Solid Edge part; units mm, degrees
sketch "Sketch1" plane through (0, 0, 0) normal (0, 0, 1) x (1, 0, 0)
  circle A0 centre (0, 0) radius 3.5
extrude "Protrusion1" add sketch "Sketch1" along normal blind 4
sketch "Sketch2" plane through (0, 0, 0) normal (0, 0, -1) x (1, 0, 0)
  circle A0 centre (0, 0) radius 2
extrude "Protrusion2" add sketch "Sketch2" along normal blind 45
sketch "Sketch3" plane through (0, 0, -45) normal (0, 0, -1) x (1, 0, 0)
  circle A0 centre (0, 0) radius 1.9997
extrude "Cutout1" cut sketch "Sketch3" against normal blind 20 flip side to cut
chamfer "Chamfer_1" distance 0.3 angle 45 1 edges at (-1.9997, 0, -45)
sketch "Sketch4" plane through (0, 0, 4) normal (0, 0, 1) x (1, 0, 0)
  line L0 (-0.866, 1.5) -> (0.866, 1.5)
  line L1 (1.7321, 0) -> (0.866, 1.5)
  line L2 (0.866, -1.5) -> (1.7321, 0)
  line L3 (-0.866, -1.5) -> (0.866, -1.5)
  line L4 (-1.7321, 0) -> (-0.866, -1.5)
  line L5 (-0.866, 1.5) -> (-1.7321, 0)
extrude "Cutout2" cut sketch "Sketch4" against normal blind 2
properties part number "185696" material "Stainless Steel, 304"
Part model, mm, in its own coordinate system. A direction names the side the tool comes from. Coordinates: 2 decimals unless noted, no trailing zeros. Write each loop counter-clockwise with the first axis right and the second up, starting at its lowest first coordinate (ties: lowest second). Pieces come first, ordered by that corner, then holes.
Item 1: Slice it at D-D (x = 2.5). Write the cut outline in (y, z).
Item 2: Mould opens along X. For faces 4 (the face through (2, -2, 0)), 5 (the face through (0, -2, -12)), 6 (the face through (-1.305, -0.74, 3.014)) say: released by +X, released by -X, zero draft, split by the parting line, or undercut.
Item 3: Probe line 1 (Z direction, x = 2, y = 2.5); line 2 (Z direction, x = -0.25, y = 1); line 3 (Y direction, x = 0, z = -4.5). List the from-to ranges inside material, lowest first.
Item 4: Pin check, flat tip, straight feed: pin 1 (3 mm diameter, centred on y = -1.5, z = -16, fed in from -X). Stop position of the tip, or through.
Item 5: Which spindle directions (+Z, -Z, +X, -X, +Y, -Y) get a long thin tool onto all of the face, cutting with end or side? Do faces 1 (the face through (0, 0, -45)), 2 (the face through (0.923, 1.774, -34.988)), 3 (the face through (1.293, -0.76, 3.014)). Say none if no direction does.
Item 6: Slice it at B-B (z = -7.5). Write the cut outline in (x, y).
Results found:
1. outline: (-2.45, 0) - (2.45, 0) - (2.45, 4) - (-2.45, 4) - close
2. face 4: zero draft
2. face 5: split by the parting line
2. face 6: undercut
3. line 1: z = 0 to 4
3. line 2: z = -45 to 2
3. line 3: y = -2 to 2
4. pin 1: stops at x = -2
5. face 1: -Z, +X, -X, +Y, -Y
5. face 2: -Z
5. face 3: +Z
6. outline: circle Ø4 at (0, 0)
